```python
from build123d import *

# Parameters (mm, degrees)
F1_DEPTH  = 25
F2_DEPTH  = 77.880271
F1_FACE_W = 69.874778
F1_FACE_H = 25
F3_DEPTH  = 43.570839


with BuildPart() as f1:
    # F0 (on Top) → F1 (new body)
    with BuildSketch(Plane.XY):
        with BuildLine():
            Line((96.185938, -34.937389), (96.185938, 34.937389))
            Line((96.185938, 34.937389), (46.22232, 34.937389))
            ThreePointArc((46.22232, 34.937389), (70.926784, 24.704465), (81.159709, 0))
            ThreePointArc((81.159709, 0), (70.926784, -24.704465), (46.22232, -34.937389))
            Line((46.22232, -34.937389), (96.185938, -34.937389))
        make_face()
        with BuildLine():
            Line((46.22232, -34.937389), (46.22232, 34.937389))
            ThreePointArc((46.22232, 34.937389), (11.28493, 0), (46.22232, -34.937389))
        make_face()
        with BuildLine():
            ThreePointArc((81.159709, 0), (70.926784, 24.704465), (46.22232, 34.937389))
            Line((46.22232, 34.937389), (46.22232, -34.937389))
            ThreePointArc((46.22232, -34.937389), (70.926784, -24.704465), (81.159709, 0))
        make_face()
    extrude(amount=F1_DEPTH)

    # F0 (on Top) → F2 (join)
    with BuildSketch(Plane.XY):
        with BuildLine():
            ThreePointArc((81.159709, 0), (70.926784, 24.704465), (46.22232, 34.937389))
            Line((46.22232, 34.937389), (46.22232, -34.937389))
            ThreePointArc((46.22232, -34.937389), (70.926784, -24.704465), (81.159709, 0))
        make_face()
        with BuildLine():
            Line((46.22232, -34.937389), (46.22232, 34.937389))
            ThreePointArc((46.22232, 34.937389), (11.28493, 0), (46.22232, -34.937389))
        make_face()
    extrude(amount=F2_DEPTH)

    # F1_face (on face) → F3 (join)
    with BuildSketch(Plane(origin=(96.185938, 0, 12.5), x_dir=(0, 1, 0), z_dir=(1, 0, 0))):
        Rectangle(F1_FACE_W, F1_FACE_H)
    extrude(amount=F3_DEPTH)


solid = f1.part
```
Here's how the part is built. I have some questions about the finished solid (model axes, mm). Coordinates: 2 decimals unless noted, no trailing zeros. Loops run counter-clockwise (first coordinate to the right, second up) from the corner with the lowest first, then second, coordinate; pieces in that order, holes last. Notation, with made-up numbers: M 4.5,53.25 L 52.5,53.25 A25 ccw 52.5,68.25 Z; hole C 21.5,26.25 d7. An arc over 180 degrees is marked long. One line per item, written item: value.
1. Imagine slicing it at B-B (x = 107.5). List the corners of the cut face in (y, z) for me, and give its area (3 significant figures).
Geometry says:
outline: M -34.94,0 L 34.94,0 L 34.94,25 L -34.94,25 Z
area: 1,750 mm2
2. Imagine slicing it at A-A (z = 19.5). List the corners of the cut face in (x, y) for me, and give its area (3 significant figures).
Geometry says:
outline: M 46.22,-34.94 L 139.76,-34.94 L 139.76,34.94 L 46.22,34.94 A34.94 ccw Z
area: 8,450 mm2
3. Will these pins go through, and if not, where does the flat tip stop? pin 1 Ø5 at (y, z) = (-17.5, 68) entering from -X; pin 2 Ø4 at (y, z) = (26.5, 52.5) entering from -X; pin 3 Ø6 at (y, z) = (-9.5, 52.5) entering from +X.
Geometry says:
pin 1: stops at x = 14.67
pin 2: stops at x = 21.32
pin 3: stops at x = 80.55
4. Imagine slicing it at C-C (y = -18). List the corners of the cut face in (x, z) for me, and give its area (3 significant figures).
Geometry says:
outline: M 16.28,0 L 139.76,0 L 139.76,25 L 76.17,25 L 76.17,77.88 L 16.28,77.88 Z
area: 6,250 mm2
5. Please list where these lines run through material, in increasing order: probe 1 along X at (y, z) = (-1, 54); probe 2 along Z at (x, y) = (67, -30); probe 3 along Y at (x, z) = (47.5, 72.5).
Geometry says:
probe 1: x = 11.3 to 81.15
probe 2: z = 0 to 25
probe 3: y = -34.91 to 34.91
6. Imagine slicing it at D-D (y = 23.5). List the corners of the cut face in (x, z) for me, and give its area (3 significant figures).
Geometry says:
outline: M 20.37,0 L 139.76,0 L 139.76,25 L 72.08,25 L 72.08,77.88 L 20.37,77.88 Z
area: 5,720 mm2
